```python
from build123d import *

# Parameters (mm, degrees)
SKETCH1_R           = 4
SKETCH1_R_2         = 4.136999592
BOSS_EXTRUDE1_DEPTH = 5.08


with BuildPart() as part:
    # Sketch1 → Boss-Extrude1 (new body)
    with BuildSketch(Plane.XY):
        with BuildLine():
            Line((-6.133755041, -250.411017633), (-6.133755041, -263.111017633))
            Line((-6.133755041, -263.111017633), (6.566244959, -263.111017633))
            Line((6.566244959, -263.111017633), (6.566244959, -258.031017633))
            Line((6.566244959, -258.031017633), (56.490143771, -258.031017633))
            Line((56.490143771, -258.031017633), (56.490143771, -263.111017633))
            Line((56.490143771, -263.111017633), (69.190143771, -263.111017633))
            ThreePointArc((69.190143771, -263.111017633), (45.84381153, -148.493633523), (69.190143771, -33.876249413))
            Line((69.190143771, -33.876249413), (56.490143771, -33.876249413))
            Line((56.490143771, -33.876249413), (56.490143771, -38.956249413))
            Line((56.490143771, -38.956249413), (6.566244959, -38.956249413))
            Line((6.566244959, -38.956249413), (6.566244959, -33.876249413))
            Line((6.566244959, -33.876249413), (-6.133755041, -33.876249413))
            Line((-6.133755041, -33.876249413), (-6.133755041, -46.576249413))
            Line((-6.133755041, -46.576249413), (-1.053755041, -46.576249413))
            Line((-1.053755041, -46.576249413), (-1.053755041, -250.411017633))
            Line((-1.053755041, -250.411017633), (-6.133755041, -250.411017633))
        make_face()
        with Locations((47.132064803, -58.435465331)):
            Circle(SKETCH1_R, mode=Mode.SUBTRACT)
        with Locations((51.42519067, -241.419788328)):
            Circle(SKETCH1_R_2, mode=Mode.SUBTRACT)
    extrude(amount=BOSS_EXTRUDE1_DEPTH)


solid = part.part
```
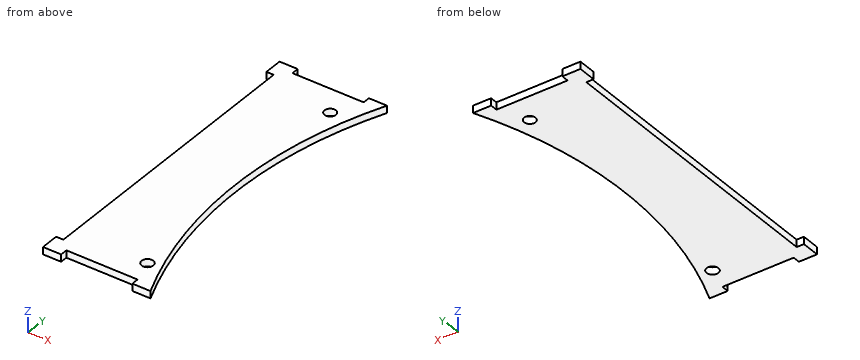
Input: part model. Units: mm. Frame: model coordinates. Coordinates: 2 decimals unless noted, no trailing zeros. Write each loop counter-clockwise with the first axis right and the second up, starting at its lowest first coordinate (ties: lowest second). Pieces come first, ordered by that corner, then holes. Notation, with made-up numbers: (-11.75, 51) -> (46.25, 51) arc R26 cw to (46.25, 77) -> close; hole circle Ø4 at (28.5, 76). An arc over 180 degrees is marked (long way). Write each question's results on one line, items separated by ' | '.
Item 1: Pin query (flat end, axial travel): pin 1 Ø2.5 at (y, z) = (-260, 2) entering from +X; pin 2 Ø1 at (y, z) = (-177.5, 2) entering from -X. Return the tip coordinate at first contact, or that it passes through.
Conclusion:
pin 1: stops at x = 68.41 | pin 2: stops at x = -1.05
Item 2: Section query B-B on z = 0.9. Return loops of the section in (x, y).
Conclusion:
outline: (-6.13, -263.11) -> (6.57, -263.11) -> (6.57, -258.03) -> (56.49, -258.03) -> (56.49, -263.11) -> (69.19, -263.11) arc R293.03 cw to (69.19, -33.88) -> (56.49, -33.88) -> (56.49, -38.96) -> (6.57, -38.96) -> (6.57, -33.88) -> (-6.13, -33.88) -> (-6.13, -46.58) -> (-1.05, -46.58) -> (-1.05, -250.41) -> (-6.13, -250.41) -> close; hole circle Ø8 at (47.13, -58.44); hole circle Ø8.27 at (51.43, -241.42)
Item 3: Material intervals for probe 1 along Y at (x, z) = (18.5, 3.7); probe 2 along X at (y, z) = (-217, 4.05); probe 3 along X at (y, z) = (-186.5, 2.75), sorted ascending.
Conclusion:
probe 1: y = -258.03 to -38.96 | probe 2: x = -1.05 to 53.96 | probe 3: x = -1.05 to 48.32
Item 4: Section query D-D on y = -228. Return loops of the section in (x, z).
Conclusion:
outline: (-1.05, 0) -> (56.84, 0) -> (56.84, 5.08) -> (-1.05, 5.08) -> close
Item 5: Section query C-C on x = 30.5. Return loops of the section in (y, z).
Conclusion:
outline: (-258.03, 0) -> (-38.96, 0) -> (-38.96, 5.08) -> (-258.03, 5.08) -> close
Item 6: Section query A-A on x = 63. Return loops of the section in (y, z).
Conclusion:
outline: (-263.11, 0) -> (-247.29, 0) -> (-247.29, 5.08) -> (-263.11, 5.08) -> close; (-49.7, 0) -> (-33.88, 0) -> (-33.88, 5.08) -> (-49.7, 5.08) -> close
